Geometry check sheet. Reference: the model listing, model coordinates, mm. Coordinates: 2 decimals unless noted, no trailing zeros. Write each loop counter-clockwise with the first axis right and the second up, starting at its lowest first coordinate (ties: lowest second). Pieces come first, ordered by that corner, then holes. Notation, with made-up numbers: (-34.75, -11.5) -> (7.25, -11.5) arc R11 cw to (7.25, -6.5) -> close; hole circle Ø7 at (24.25, 1). An arc over 180 degrees is marked (long way). One line per question, with ' | ' between items.
```python
from build123d import *
from OCP.BRepFilletAPI import BRepFilletAPI_MakeChamfer

# Parameters (mm, degrees)
CHAMFER1_SIZE  = 0.254
CHAMFER1_SIZE2 = 0.213389286
FILLET1_R      = 0.508


with BuildPart() as part:
    # Sketch1 → Revolve1 (revolve)
    with BuildSketch(Plane(origin=(0, 0, 0), x_dir=(0, 0, -1), z_dir=(1, 0, 0)), mode=Mode.PRIVATE) as revolve1_sk:
        with BuildLine():
            Line((32.131, 15.875), (32.131, 8.128))
            Line((32.131, 8.128), (37.222917887, 8.128))
            ThreePointArc((37.222917887, 8.128), (36.1372367, 12.071044848), (34.635160964, 15.875))
            Line((34.635160964, 15.875), (32.131, 15.875))
        make_face()
    revolve(revolve1_sk.sketch.rotate(Axis((0, 0, 0), (0, 0, -1)), 90), axis=Axis((0, 0, 0), (0, 0, -1)))

    # Chamfer1: one chamfer whose edges measure the first distance from different faces: ONE call of the kernel's chamfer builder (chamfer() names one face for all edges)
    chamfer1_edges_1 = [part.edges().sort_by_distance(p)[0] for p in [
        (-8.128, 0, -37.222917887),
    ]]
    chamfer1_side_1 = [part.faces().sort_by_distance(p)[0] for p in [
        (-8.128, 0, -34.676958943),
    ]]
    chamfer1_edges_2 = [part.edges().sort_by_distance(p)[0] for p in [
        (-8.128, 0, -32.131),
    ]]
    chamfer1 = BRepFilletAPI_MakeChamfer(part.part.solid().wrapped)
    for e in chamfer1_edges_1:
        chamfer1.Add(CHAMFER1_SIZE, CHAMFER1_SIZE2, e.wrapped, chamfer1_side_1[0].wrapped)  # the first distance lies on this face
    for e in chamfer1_edges_2:
        chamfer1.Add(CHAMFER1_SIZE, e.wrapped)
    add(Compound.cast(chamfer1.Shape()), mode=Mode.REPLACE)

    # Fillet1
    fillet1_edges = [part.edges().sort_by_distance(p)[0] for p in [
        (-15.875, 0, -34.635160964),
        (-15.875, 0, -32.131),
    ]]
    fillet(fillet1_edges, radius=FILLET1_R)


solid = part.part
```
(1) Cross-section at B-B (z = -35.3). Record the cut outline in (x, y), plus the area to 3 significant figures.
Answers below:
outline: circle Ø28.67 at (0, 0); hole circle Ø16.26 at (0, 0) | area: 438 mm²
(2) Cross-section at A-A (z = -33.6). Record the cut outline in (x, y) (3 decimals).
Answers below:
outline: circle Ø31.75 at (0, 0); hole circle Ø16.256 at (0, 0)
(3) Depth check by flat-ended pin: P1, Ø2, axis at x = -3.5, y = 10.5, coming from the -Z side; P2, Ø1.5, axis at x = -12.5, y = 10.5, coming from the +Z side. Enter the tip coordinate at first touch or a pass-through.
Answers below:
P1: stops at z = -36.75 | P2: stops at z = -32.18
(4) Material ranges on line 1 (Y direction, x = 0, z = -33.4) (3 decimals); line 2 (Y direction, x = 6.5, z = -33.4), recorded low to high.
Answers below:
line 1: y = -15.875 to -8.128, 8.128 to 15.875 | line 2: y = -14.48 to -4.88, 4.88 to 14.48
(5) Draft check along X on faces 1 (the face through (7, 7, -32.131)), 2 (the face through (15.14, -4.77, -33.46)), 3 (the face through (-1.762, 7.935, -34.709)). Enter one of: pulls with the +X half, pulls with the -X half, needs draft (parallel to the pull), parting line crosses it, or undercut.
Answers below:
face 1: needs draft | face 2: parting line crosses it | face 3: undercut
